Could you check a few things on this model? Use its own coordinates, in mm. Face numbers are marked on the shaded views. A direction names the side the tool comes from. Round coordinates to 2 decimals unless told otherwise and drop trailing zeros. Loops run counter-clockwise (first coordinate to the right, second up) from the corner with the lowest first, then second, coordinate; pieces in that order, holes last. Notation, with made-up numbers: M 20,-37.75 L 76,-37.75 A9 cw 76,-23.75 Z; hole C 73,31.25 d5. An arc over 180 degrees is marked long. One line per item, written item: value. Start each with the question number.
Q1. Which directions (+Z, -Z, +X, -X, +Y, -Y) give clear straight access to the entire face, cutting with the end or side of a thin tool? Please do the marked faces 1 and 2.
Q2. Thinking about a two-plate mould opening in Y: for the marked faces 3, 4 and 5, which applies, released by +Y, released by -Y, zero draft, split by the parting line, or undercut?
Q3. Imagine slicing it at C-C (y = -9). Please give me the cut outline in (x, z).
Q4. I'm going to push flat-ended pins straight in: pin 1 Ø2 at (y, z) = (-5.5, 13.5) entering from +X; pin 2 Ø6 at (x, y) = (17, -7.5) entering from -Z. Where does each tip first touch, or does it pass through?
Q5. Please list where these lines run through material, in increasing order: line 1 along Z through (x, y) = (4.25, -8); line 2 along Z through (x, y) = (18.5, -7); line 3 along X through (y, z) = (-1, 23.5).
from build123d import *

# Parameters (mm, degrees)
F1_DEPTH = 10
F2_R     = 4.99999


# Not quite as in the source:
# - a fillet or chamfer is up to 0.001 mm smaller than in the source, because OpenCascade refuses the exact size


with BuildPart() as f1:
    # F0 (on Front) → F1 (new body)
    with BuildSketch(Plane.XZ):
        Polygon((0, 30), (0, 0), (10, 0), (10, 20), (20, 20), (20, 30), align=None)
    extrude(amount=F1_DEPTH)

    # F2 (radius 5 in the source; OpenCascade refuses exactly that, so slightly less here)
    f2_edges = [f1.edges().sort_by_distance(p)[0] for p in [
        (10, -10, 30),
        (10, 0, 30),
        (0, -10, 15),
        (10, -10, 10),
        (15, -10, 20),
        (10, 0, 10),
        (15, 0, 20),
        (0, 0, 15),
    ]]
    fillet(f2_edges, radius=F2_R)


solid = f1.part
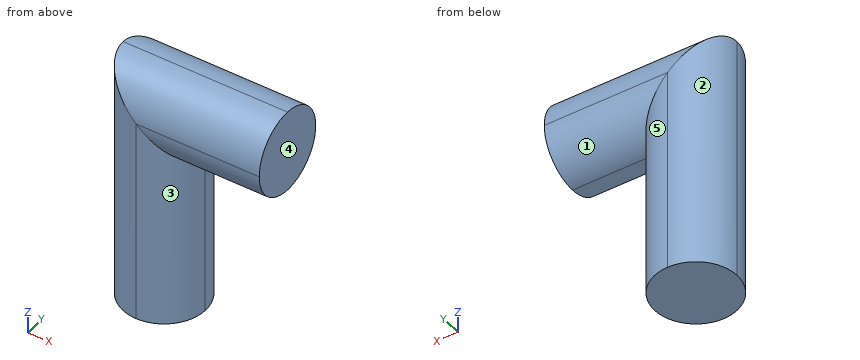
Report:
1. face 1: -Z, +X, +Y
1. face 2: +Z, -Z, -X, +Y
2. face 3: released by -Y
2. face 4: zero draft
2. face 5: released by +Y
3. outline: M 2,0 L 8,0 L 8,22 L 20,22 L 20,28 L 2,28 Z
4. pin 1: stops at x = 10
4. pin 2: stops at z = 20
5. line 1: z = 0 to 29
5. line 2: z = 20.42 to 29.58
5. line 3: x = 2 to 20
